Work out the finished part from the listing and answer in its coordinate system (mm). Face numbers are marked on the shaded views. A direction names the side the tool comes from. Give positions to 0.01 mm unless a question says otherwise; leave off trailing zeros. Write each question's results on one line, items separated by ' | '. Start each with the question number.
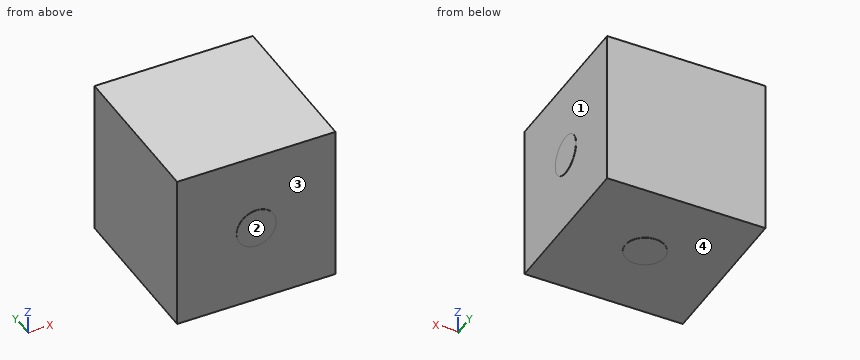
from build123d import *

# Parameters (mm, degrees)
F0_W     = 152.4
F0_H     = 152.4
F1_DEPTH = 152.4
F2_R     = 19.05
F3_DEPTH = 0.254
F4_R     = 19.05
F5_DEPTH = 0.254
F6_R     = 19.05
F7_DEPTH = 0.254


with BuildPart() as f1:
    # F0 (on Top) → F1 (new body)
    with BuildSketch(Plane.XY):
        with Locations((76.2, -76.2)):
            Rectangle(F0_W, F0_H)
    extrude(amount=F1_DEPTH)

    # F2 (on face) → F3 (join)
    with BuildSketch(Plane.XZ.offset(152.4)):
        with Locations((76.2, 76.2)):
            Circle(F2_R)
    extrude(amount=F3_DEPTH)

    # F4 (on face) → F5 (join)
    with BuildSketch(Plane.YZ.offset(152.4)):
        with Locations((-76.2, 76.2)):
            Circle(F4_R)
    extrude(amount=F5_DEPTH)

    # F6 (on face) → F7 (join)
    with BuildSketch(Plane(origin=(0, 0, 0), x_dir=(1, 0, 0), z_dir=(0, 0, -1))):
        with Locations((76.2, 76.2)):
            Circle(F6_R)
    extrude(amount=F7_DEPTH)


solid = f1.part
Q1. Consider L1, parallel to Z at x = 55, y = -139.5; L2, parallel to Y at x = 124.5, z = 17. Determine where each line is inside the solid, lowest interval first.
Q2. A tool of negligible diameter and unlimited length cuts with its end or side. For the marked faces 1, 2, 3 and 4, from which of +Z, -Z, +X, -X, +Y, -Y can it reach the whole face along a straight path? Write none if from no direction.
Q3. Given pin 1 (10 mm diameter, centred on x = 110.5, y = -83.5, fed in from -Z); pin 2 (5 mm diameter, centred on y = -106.5, z = 59.5, fed in from +X), each flat-ended and moving along its own axis, determine where each tip first touches the part or whether it passes through.
Result:
1) L1: z = 0 to 152.4 | L2: y = -152.4 to 0
2) face 1: +X | face 2: +Z, -Z, +X, -X, -Y | face 3: -Y | face 4: -Z
3) pin 1: stops at z = 0 | pin 2: stops at x = 152.4
